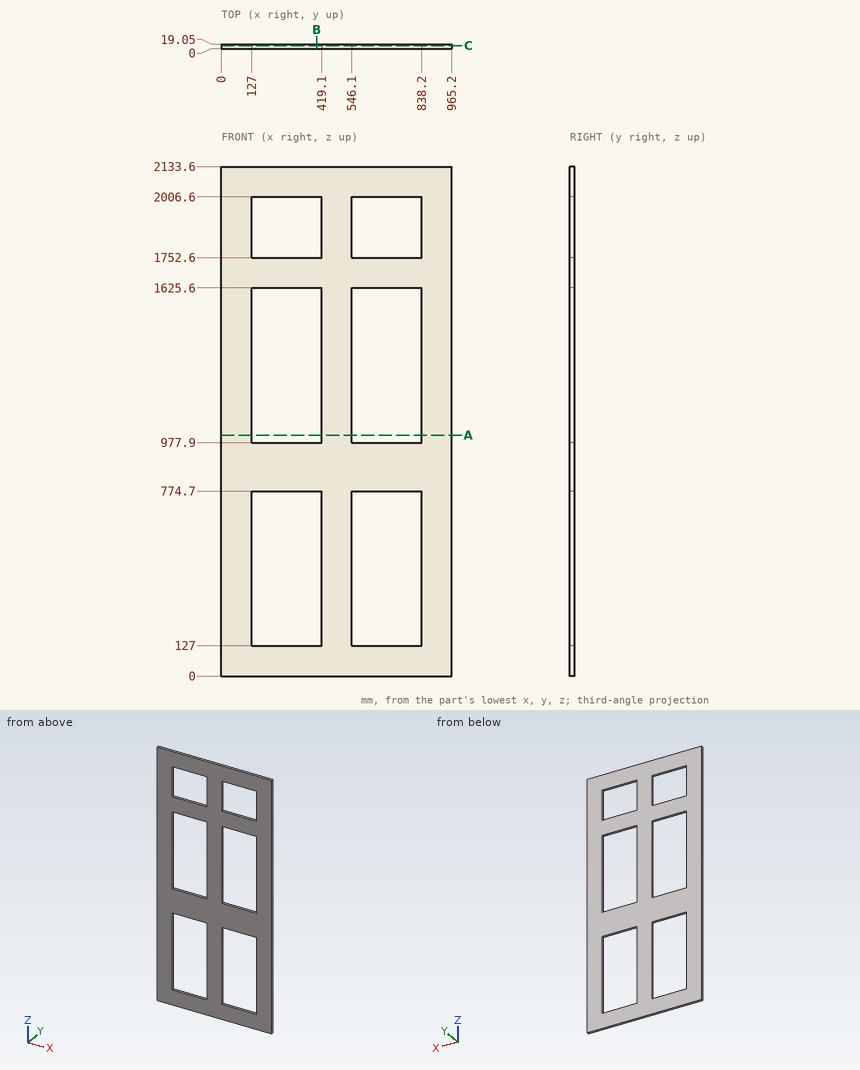
Can you work these out from the drawing? Everything is in mm from the part's minimum corner. Round coordinates to 2 decimals unless told otherwise and drop trailing zeros. Write each loop counter-clockwise with the first axis right and the second up, starting at its lowest first coordinate (ties: lowest second). Pieces come first, ordered by that corner, then holes.
1. Suppose I cut it at C-C (y = 11.75). List the corners of the cut face in (x, z) for me, and give its area (3 significant figures).
2. Suppose I cut it at A-A (z = 1008.5). List the corners of the cut face in (x, y) for me.
3. Suppose I cut it at B-B (x = 398.5). List the corners of the cut face in (y, z) for me.
4. Will this pin go through, and if not, where does the flat tip stop? pin 1 Ø5 at (y, z) = (11, 245.5) entering from -X.
5. I need wall thicknesses on L1, parallel to X at y = 18, z = 1599.5; L2, parallel to Z at x = 707.5, y = 5.5. Which ranges of each line are inside material? Lowest first, please.
Answer sheet:
1. outline: (0, 0) - (965.2, 0) - (965.2, 2133.6) - (0, 2133.6) - close; hole (127, 127) - (419.1, 127) - (419.1, 774.7) - (127, 774.7) - close; hole (127, 977.9) - (419.1, 977.9) - (419.1, 1625.6) - (127, 1625.6) - close; hole (127, 1752.6) - (419.1, 1752.6) - (419.1, 2006.6) - (127, 2006.6) - close; hole (546.1, 127) - (838.2, 127) - (838.2, 774.7) - (546.1, 774.7) - close; hole (546.1, 977.9) - (838.2, 977.9) - (838.2, 1625.6) - (546.1, 1625.6) - close; hole (546.1, 1752.6) - (838.2, 1752.6) - (838.2, 2006.6) - (546.1, 2006.6) - close
1. area: 1,150,000 mm2
2. outline: (0, 0) - (127, 0) - (127, 19.05) - (0, 19.05) - close; (419.1, 0) - (546.1, 0) - (546.1, 19.05) - (419.1, 19.05) - close; (838.2, 0) - (965.2, 0) - (965.2, 19.05) - (838.2, 19.05) - close
3. outline: (0, 0) - (19.05, 0) - (19.05, 127) - (0, 127) - close; (0, 774.7) - (19.05, 774.7) - (19.05, 977.9) - (0, 977.9) - close; (0, 1625.6) - (19.05, 1625.6) - (19.05, 1752.6) - (0, 1752.6) - close; (0, 2006.6) - (19.05, 2006.6) - (19.05, 2133.6) - (0, 2133.6) - close
4. pin 1: stops at x = 0
5. L1: x = 0 to 127, 419.1 to 546.1, 838.2 to 965.2
5. L2: z = 0 to 127, 774.7 to 977.9, 1625.6 to 1752.6, 2006.6 to 2133.6
